Verification items for the finished model (mm, model axes). A direction names the side the tool comes from. Give positions to 0.01 mm unless a question says otherwise; leave off trailing zeros. Loops run counter-clockwise (first coordinate to the right, second up) from the corner with the lowest first, then second, coordinate; pieces in that order, holes last. Notation, with made-up numbers: M 52,-21.75 L 111,-21.75 A25 ccw 111,3.25 Z; hole C 79.25,17 d5. An arc over 180 degrees is marked long. Use a Markdown table: item, result.
from build123d import *

# Parameters (mm, degrees)
SKETCH1_W           = 57
SKETCH1_H           = 33
BOSS_EXTRUDE1_DEPTH = 10
SKETCH3_R           = 3.35
CUT_EXTRUDE1_DEPTH  = 11
SKETCH4_R           = 3.35
CUT_EXTRUDE2_DEPTH  = 11
SKETCH10_R          = 3.35
CUT_EXTRUDE5_DEPTH  = 11
SKETCH12_R          = 3.35
CUT_EXTRUDE6_DEPTH  = 11
SKETCH16_W          = 57
SKETCH16_H          = 4
CUT_EXTRUDE7_DEPTH  = 4
SKETCH17_R          = 10
CUT_EXTRUDE8_DEPTH  = 6


with BuildPart() as part:
    # Sketch1 → Boss-Extrude1 (new body)
    with BuildSketch(Plane(origin=(0, 0, 0), x_dir=(1, 0, 0), z_dir=(0, 1, 0))):
        with Locations((28.5, 16.5)):
            Rectangle(SKETCH1_W, SKETCH1_H)
    extrude(amount=BOSS_EXTRUDE1_DEPTH)

    # Sketch3 → Cut-Extrude1 (cut, through all)
    with BuildSketch(Plane.XZ):
        with Locations((6, -6.5)):
            Circle(SKETCH3_R)
    extrude(amount=-CUT_EXTRUDE1_DEPTH, mode=Mode.SUBTRACT)

    # Sketch4 → Cut-Extrude2 (cut, through all)
    with BuildSketch(Plane.XZ):
        with Locations((51, -26.5)):
            Circle(SKETCH4_R)
    extrude(amount=-CUT_EXTRUDE2_DEPTH, mode=Mode.SUBTRACT)

    # Sketch10 → Cut-Extrude5 (cut, through all)
    with BuildSketch(Plane.XZ):
        with Locations((6, -26.5)):
            Circle(SKETCH10_R)
    extrude(amount=-CUT_EXTRUDE5_DEPTH, mode=Mode.SUBTRACT)

    # Sketch12 → Cut-Extrude6 (cut, through all)
    with BuildSketch(Plane.XZ):
        with Locations((51, -6.5)):
            Circle(SKETCH12_R)
    extrude(amount=-CUT_EXTRUDE6_DEPTH, mode=Mode.SUBTRACT)

    # Sketch16 → Cut-Extrude7 (cut)
    with BuildSketch(Plane(origin=(0, 10, 0), x_dir=(1, 0, 0), z_dir=(0, 1, 0))):
        with Locations((28.5, 16.5)):
            Rectangle(SKETCH16_W, SKETCH16_H)
    extrude(amount=-CUT_EXTRUDE7_DEPTH, mode=Mode.SUBTRACT)

    # Sketch17 → Cut-Extrude8 (cut)
    with BuildSketch(Plane(origin=(0, 10, 0), x_dir=(1, 0, 0), z_dir=(0, 1, 0))):
        with Locations((28.5, 16.5)):
            Circle(SKETCH17_R)
    extrude(amount=-CUT_EXTRUDE8_DEPTH, mode=Mode.SUBTRACT)


solid = part.part
(1) Gauge pin test, flat ends, axial feed: P1, Ø4, axis at y = 1.5, z = -28, coming from the -X side; P2, Ø2, axis at x = 43, z = -16, coming from the +Y side; P3, Ø6, axis at x = 51, z = -6.5, coming from the +Y side; P4, Ø10, axis at x = 30, z = -19, coming from the +Y side. Record the tip position at first contact, or that the pin passes through.
Results below:
| item | result |
|---|---|
| P1 | x = 0 |
| P2 | y = 6 |
| P3 | through |
| P4 | y = 4 |
(2) Set-up check for faces 1 (the flat face through (28, 4, -17)), 2 (the flat face through (28, 10, -27)), 3 (the flat face through (9, 6, -17)): record each of +Z, -Z, +X, -X, +Y, -Y from which the full face is reachable in a straight line by a thin tool's end or side.
Results below:
| item | result |
|---|---|
| face 1 | +Y |
| face 2 | +Z, -Z, +X, -X, +Y |
| face 3 | +X, -X, +Y |
(3) Cross-section at B-B on x = 6. Record the cut outline in (y, z).
Results below:
| item | result |
|---|---|
| outline | M 0,-33 L 10,-33 L 10,-29.85 L 0,-29.85 Z; M 0,-23.15 L 10,-23.15 L 10,-18.5 L 6,-18.5 L 6,-14.5 L 10,-14.5 L 10,-9.85 L 0,-9.85 Z; M 0,-3.15 L 10,-3.15 L 10,0 L 0,0 Z |
(4) Draft check along X on faces 4 (the flat face through (57, 5, -16)), 5 (the flat face through (9, 8, -14.5)), 6 (the cylindrical face through (38.04, 7.04, -19.5)). Enter one of: +X half, -X half, draft (parallel to the pull), parting line (faces both ways), or undercut.
Results below:
| item | result |
|---|---|
| face 4 | +X half |
| face 5 | draft |
| face 6 | undercut |
(5) Cross-section at D-D on z = -16.5. Record the cut outline in (x, y).
Results below:
| item | result |
|---|---|
| outline | M 0,0 L 57,0 L 57,6 L 38.5,6 L 38.5,4 L 18.5,4 L 18.5,6 L 0,6 Z |
(6) Cross-section at A-A on y = 8.25. Record the cut outline in (x, z).
Results below:
| item | result |
|---|---|
| outline | M 0,-33 L 57,-33 L 57,-18.5 L 38.3,-18.5 A10 cw 18.7,-18.5 L 0,-18.5 Z; M 0,-14.5 L 18.7,-14.5 A10 cw 38.3,-14.5 L 57,-14.5 L 57,0 L 0,0 Z; hole C 6,-26.5 d6.7; hole C 6,-6.5 d6.7; hole C 51,-26.5 d6.7; hole C 51,-6.5 d6.7 |
(7) Material ranges on line 1 (Z direction, x = 51, y = 7); line 2 (Z direction, x = 51, y = 4); line 3 (Z direction, x = 28.5, y = 6.2), recorded low to high.
Results below:
| item | result |
|---|---|
| line 1 | -33 to -29.85, -23.15 to -18.5, -14.5 to -9.85, -3.15 to 0 |
| line 2 | -33 to -29.85, -23.15 to -9.85, -3.15 to 0 |
| line 3 | -33 to -26.5, -6.5 to 0 |
(8) Cross-section at C-C on y = 2.5. Record the cut outline in (x, z).
Results below:
| item | result |
|---|---|
| outline | M 0,-33 L 57,-33 L 57,0 L 0,0 Z; hole C 6,-26.5 d6.7; hole C 6,-6.5 d6.7; hole C 51,-26.5 d6.7; hole C 51,-6.5 d6.7 |
